Geometry check sheet. Reference: the model listing, model coordinates, mm. Face numbers are marked on the shaded views. A direction names the side the tool comes from. Coordinates: 2 decimals unless noted, no trailing zeros. Write each loop counter-clockwise with the first axis right and the second up, starting at its lowest first coordinate (ties: lowest second). Pieces come first, ordered by that corner, then holes. Notation, with made-up numbers: (-7.5, 88) -> (37.5, 88) arc R16 ccw to (37.5, 112) -> close; hole circle Ø10 at (-9, 1). An arc over 180 degrees is marked (long way). One line per question, with ' | ' between items.
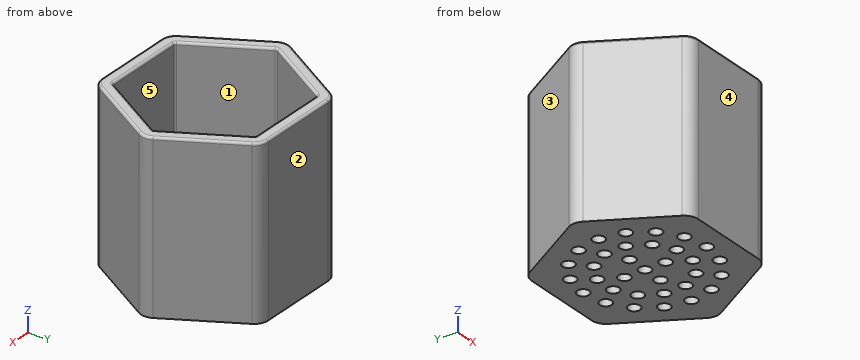
```python
from build123d import *

# Parameters (mm, degrees)
F1_DEPTH        = 70
F3_DEPTH        = 5
F4_R            = 2.5
F5_DEPTH        = 5
F5_COPIES_COUNT = 4
F7_R            = 2.5
F8_DEPTH        = 5
F9_R            = 6
F10_R           = 1
F11_R           = 1


# Not quite as in the source:
# - a pattern or mirror of a feature is missing from the dataset's text; its kind, count and spacing are read off the source's solid


with BuildPart() as f1:
    # F0 (on Top) → F1 (new body)
    with BuildSketch(Plane.XY):
        Polygon((20.2072594216, 35), (-20.2072594216, 35), (-40.4145188433, 0), (-20.2072594216, -35), (20.2072594216, -35), (40.4145188433, 0), align=None)
        Polygon((-17.3205080757, -30), (-34.6410161514, 0), (-17.3205080757, 30), (17.3205080757, 30), (34.6410161514, 0), (17.3205080757, -30), align=None, mode=Mode.SUBTRACT)
    extrude(amount=F1_DEPTH)

    # F2 (on face) → F3 (join)
    with BuildSketch(Plane(origin=(0, 0, 0), x_dir=(1, 0, 0), z_dir=(0, 0, -1))):
        Polygon((-20.2072594216, 35), (-40.4145188433, 0), (-20.2072594216, -35), (20.2072594216, -35), (40.4145188433, 0), (20.2072594216, 35), align=None)
    extrude(amount=-F3_DEPTH)

    # F4 (on face) → F5 (cut, through all)
    with BuildSketch(Plane.XY.offset(5)):
        with Locations((0, 26)):
            Circle(F4_R)
        with Locations((4.4861967818, 16.7427143223)):
            Circle(F4_R)
        with Locations((0, 8.6666666667)):
            Circle(F4_R)
        with Locations((12.2565175406, 12.2565175406)):
            Circle(F4_R)
        with Locations((9.9497692415, 24.0208678453)):
            Circle(F4_R)
        with Locations((24.0208678453, 9.9497692415)):
            Circle(F4_R)
        with Locations((16.7427143223, 4.4861967818)):
            Circle(F4_R)
        with Locations((18.3847763109, 18.3847763109)):
            Circle(F4_R)
    f5 = extrude(amount=-F5_DEPTH, mode=Mode.SUBTRACT)

    # F5_copies: F5 ×4 about axis
    f5_copies_axis = Axis((0, 0, 0), (0, 0, 1))
    for i in range(1, F5_COPIES_COUNT):
        add(f5.rotate(f5_copies_axis, i * 360 / F5_COPIES_COUNT), mode=Mode.SUBTRACT)

    # F7 (on face) → F8 (cut, through all)
    with BuildSketch(Plane.XY.offset(5)):
        Circle(F7_R)
    extrude(amount=-F8_DEPTH, mode=Mode.SUBTRACT)

    # F9
    f9_edges = [f1.edges().sort_by_distance(p)[0] for p in [
        (-20.207259, 35, 35),
        (-40.414519, 0, 35),
        (-20.207259, -35, 35),
        (20.207259, -35, 35),
        (40.414519, 0, 35),
        (20.207259, 35, 35),
    ]]
    fillet(f9_edges, radius=F9_R)

    # F10
    f10_edges = [f1.edges().sort_by_distance(p)[0] for p in [
        (-17.320508, 30, 37.5),
        (17.320508, 30, 37.5),
        (34.641016, 0, 37.5),
        (17.320508, -30, 37.5),
        (-17.320508, -30, 37.5),
        (-34.641016, 0, 37.5),
        (-25.980762, 15, 5),
        (-25.980762, -15, 5),
        (0, -30, 5),
        (25.980762, -15, 5),
        (25.980762, 15, 5),
        (0, 30, 5),
    ]]
    fillet(f10_edges, radius=F10_R)

    # F11
    f11_edges = [f1.edges().sort_by_distance(p)[0] for p in [
        (-25.980762, -15, 70),
        (-17.243158, -29.866025, 70),
        (-34.486316, 0, 70),
        (0, -30, 70),
        (-25.980762, 15, 70),
        (17.243158, -29.866025, 70),
        (-17.243158, 29.866025, 70),
        (25.980762, -15, 70),
        (0, 30, 70),
        (34.486316, 0, 70),
        (17.243158, 29.866025, 70),
        (25.980762, 15, 70),
        (0, 35, 70),
        (19.743158, 34.196152, 70),
        (-19.743158, 34.196152, 70),
        (30.310889, 17.5, 70),
        (-30.310889, 17.5, 70),
        (39.486316, 0, 70),
        (-39.486316, 0, 70),
        (30.310889, -17.5, 70),
        (-30.310889, -17.5, 70),
        (19.743158, -34.196152, 70),
        (-19.743158, -34.196152, 70),
        (0, -35, 70),
    ]]
    fillet(f11_edges, radius=F11_R)


solid = f1.part
```
(1) Cross-section at A-A (z = 16.5). Record the cut outline in (x, y), plus the area to 3 significant figures.
Answers below:
outline: (-38.68, -3) -> (-21.94, -32) arc R6 ccw to (-16.74, -35) -> (16.74, -35) arc R6 ccw to (21.94, -32) -> (38.68, -3) arc R6 ccw to (38.68, 3) -> (21.94, 32) arc R6 ccw to (16.74, 35) -> (-16.74, 35) arc R6 ccw to (-21.94, 32) -> (-38.68, 3) arc R6 ccw to start; hole (-34.35, -0.5) -> (-17.61, -29.5) arc R1 ccw to (-16.74, -30) -> (16.74, -30) arc R1 ccw to (17.61, -29.5) -> (34.35, -0.5) arc R1 ccw to (34.35, 0.5) -> (17.61, 29.5) arc R1 ccw to (16.74, 30) -> (-16.74, 30) arc R1 ccw to (-17.61, 29.5) -> (-34.35, 0.5) arc R1 ccw to start | area: 1,110 mm²
(2) Tool access check on the marked faces 1 and 2. Record the directions out of +Z, -Z, +X, -X, +Y, -Y that give a thin tool (end or side, any length) a straight path to the whole face; none if there is none.
Answers below:
face 1: +Z | face 2: +Z, -Z, +X, -X, +Y
(3) Material ranges on line 1 (Y direction, x = 0, z = 2.3); line 2 (Y direction, x = -2.5, z = 58); line 3 (Z direction, x = -19, y = 7), recorded low to high.
Answers below:
line 1: y = -35 to -28.5, -23.5 to -11.17, -6.17 to -2.5, 2.5 to 6.17, 11.17 to 23.5, 28.5 to 35 | line 2: y = -35 to -30, 30 to 35 | line 3: z = 0 to 5
(4) Cross-section at B-B (x = 0). Count the separate pieces of the cut face and the enclosed holes in it, plus the area to 3 significant figures.
Answers below:
separate pieces: 6 | enclosed holes: 0 | area: 875 mm²
(5) Draft check along X on the marked faces 3, 4 and 5. Enter one of: pulls with the +X half, pulls with the -X half, needs draft (parallel to the pull), parting line crosses it, or undercut.
Answers below:
face 3: pulls with the -X half | face 4: needs draft | face 5: undercut
(6) Depth check by flat-ended pin: P1, Ø8, axis at x = -20.5, y = -19, coming from the -Z side; P2, Ø6, axis at x = 26, y = 0, coming from the +Z side; P3, Ø6, axis at y = 4.5, z = 26, coming from the -X side; P4, Ø2, axis at y = -11.5, z = 53.5, coming from the +X side. Enter the tip coordinate at first touch or a pass-through.
Answers below:
P1: stops at z = 0 | P2: stops at z = 5 | P3: stops at x = -39.3 | P4: stops at x = 34.35
